Source: CAD feature listing. Evaluate the final solid. Frame: model axes, mm. A direction names the side the tool comes from. Coordinates: 2 decimals unless noted, no trailing zeros. Loops run counter-clockwise (first coordinate to the right, second up) from the corner with the lowest first, then second, coordinate; pieces in that order, holes last. Notation, with made-up numbers: M -19,63 L 1,63 A14 cw 1,68 Z; hole C 26.5,2.25 d7. An arc over 180 degrees is marked long. One line per question, with ' | ' between items. Start each with the question number.
1. Access query for faces 4 (the flat face through (0, 2, 5.6)), 5 (the flat face through (0, -6, 0)), 6 (the flat face through (0, 2, -2)), 7 (the flat face through (0, 6.25, 4)), 8 (the flat face through (0, -2.75, 4)). Directions: +Z, -Z, +X, -X, +Y, -Y. A direction counts if a zero-diameter tool reaches every point of the face in a straight line with its end or side. Return the directions, or none.
2. Pin query (flat end, axial travel): P1, Ø2, axis at x = 2.5, y = -6, coming from the -Z side; P2, Ø2, axis at x = 2.5, z = 3, coming from the +Y side; P3, Ø1.6, axis at x = -1.5, y = 7.5, coming from the +Z side. Return the tip coordinate at first contact, or that it passes through.
3. Section query B-B, the plane x = -1.5. Output: boundary loops of the cut face in (y, z).
4. Mould query, pull axis X, two halves, no side actions, for faces 1 (the flat face through (5.2, 2, 2)), 2 (the cylindrical face through (2.771, -6.236, 0.74)), 3 (the flat face through (0, -4.25, -1)). Classes: pulls with the +X half, pulls with the -X half, needs draft (parallel to the pull), parting line crosses it, or undercut.
5. Ray query, probe 1 along Y at (x, z) = (2.54, 0.7); probe 2 along Y at (x, z) = (-3.75, 2.25); probe 3 along Z at (x, y) = (4, -5). Return the intervals inside material, ascending.
6. Section query A-A, the plane x = 0. Output: boundary loops of the cut face in (y, z).
7. Section query C-C, the plane z = 3.5. Output: boundary loops of the cut face in (x, y).
8. Section query D-D, the plane z = -0.75. Output: boundary loops of the cut face in (x, y), and give its area (3 significant figures).
Autodesk Inventor part; units mm, degrees
ref_plane "YZ Plane" through (0, 0, 0) normal (1, 0, 0) x (0, 1, 0)
ref_plane "XZ Plane" through (0, 0, 0) normal (0, 1, 0) x (-1, 0, 0)
ref_plane "XY Plane" through (0, 0, 0) normal (0, 0, 1) x (1, 0, 0)
sketch "スケッチ1" plane through (0, 0, 0) normal (0, 0, 1) x (1, 0, 0)
  line L0 (-5.2, -8.25) -> (5.2, -8.25)
  line L1 (5.2, -8.25) -> (5.2, 8.25)
  line L2 (5.2, 8.25) -> (-5.2, 8.25)
  line L3 (-5.2, 8.25) -> (-5.2, -8.25)
  line L4 (-5.2, -8.25) -> (5.2, 8.25) construction
  line L5 (5.2, -8.25) -> (-5.2, 8.25) construction
  circle A0 centre (0, -6.68) radius 0.5
  circle A1 centre (2.54, -6.68) radius 0.5
  circle A2 centre (-2.54, -6.68) radius 0.5
  point P0 (0, 0)
  point P1 (0, 0)
  dimension "d0" = 10.4
  dimension "d1" = 16.5
  dimension "d2" = 1
  dimension "d3" = 2.54
  dimension "d4" = 2.54
  dimension "d5" = 1.57
extrude "押し出し1" add sketch "スケッチ1" along normal blind 1.5
sketch "スケッチ2" plane through (0, 0, 1.5) normal (0, 0, 1) x (1, 0, 0)
  line L0 (-5.2, 8.25) -> (-5.2, -8.25)
  line L1 (5.2, -8.25) -> (5.2, 8.25)
  line L2 (-5.2, 6.25) -> (5.2, 6.25)
  line L3 (5.2, 6.25) -> (5.2, -2.75)
  line L4 (5.2, -2.75) -> (-5.2, -2.75)
  line L5 (-5.2, -2.75) -> (-5.2, 6.25)
  line L6 (5.2, 8.25) -> (-5.2, 8.25)
  point P0 (0, 0)
  dimension "d8" = 2
  dimension "d9" = 9
extrude "押し出し2" add sketch "スケッチ2" along normal blind 4.1 contours L2 L1 L4 L0
sketch "スケッチ3" plane through (0, 0, 0) normal (0, 0, -1) x (-1, 0, 0)
  line L0 (-5.2, 8.25) -> (5.2, 8.25)
  line L1 (5.2, 8.25) -> (5.2, -8.25)
  line L2 (-5.2, 8.25) -> (5.2, 8.25)
  line L3 (5.2, 8.25) -> (5.2, -4.25)
  line L4 (5.2, -4.25) -> (-5.2, -4.25)
  line L5 (-5.2, -4.25) -> (-5.2, 8.25)
  line L6 (5.2, -8.25) -> (-5.2, -8.25)
  point P0 (0, 0)
  dimension "d12" = 4
extrude "押し出し3" add sketch "スケッチ3" along normal blind 2
properties part number "OKI-78SR"
Taken from the geometry:
1) face 4: +Z, +X, -X, +Y, -Y | face 5: -Z, +X, -X, -Y | face 6: -Z, +X, -X, +Y, -Y | face 7: +Z, +X, -X, +Y | face 8: +Z, +X, -X, -Y
2) P1: z = 0 | P2: y = 6.25 | P3: z = 1.5
3) outline: M -8.25,0 L -4.25,0 L -4.25,-2 L 8.25,-2 L 8.25,1.5 L 6.25,1.5 L 6.25,5.6 L -2.75,5.6 L -2.75,1.5 L -8.25,1.5 Z
4) face 1: pulls with the +X half | face 2: undercut | face 3: needs draft
5) probe 1: -8.25 to -7.18, -6.18 to 8.25 | probe 2: -2.75 to 6.25 | probe 3: 0 to 1.5
6) outline: M -8.25,0 L -7.18,0 L -7.18,1.5 L -8.25,1.5 Z; M -6.18,0 L -4.25,0 L -4.25,-2 L 8.25,-2 L 8.25,1.5 L 6.25,1.5 L 6.25,5.6 L -2.75,5.6 L -2.75,1.5 L -6.18,1.5 Z
7) outline: M -5.2,-2.75 L 5.2,-2.75 L 5.2,6.25 L -5.2,6.25 Z
8) outline: M -5.2,-4.25 L 5.2,-4.25 L 5.2,8.25 L -5.2,8.25 Z | area: 130 mm^2
